Geometry check sheet. Reference: the model listing, model coordinates, mm. Face numbers are marked on the shaded views. Round coordinates to 2 decimals unless told otherwise and drop trailing zeros. Write each loop counter-clockwise with the first axis right and the second up, starting at its lowest first coordinate (ties: lowest second). Pieces come first, ordered by that corner, then holes. Notation, with made-up numbers: M -8,-3.75 L -2,-3.75 A28 cw -2,33.25 Z; hole C -23.5,15 d1. An arc over 180 degrees is marked long. Put each result on its own line as item: value. Start each with the question number.
(1) Section check D-D on y = 37. Record the cut outline in (x, z), then the cut area to 3 significant figures.
(2) Section check C-C on z = 2.7. Record the cut outline in (x, y), then the cut area to 3 significant figures.
(3) Material ranges on probe 1 along Y at (x, z) = (0, 3.95); probe 2 along X at (y, z) = (1.5, 2.4); probe 3 along X at (y, z) = (54, 0.5), recorded low to high.
(4) Section check A-A on y = 0. Record the cut outline in (x, z), then the cut area to 3 significant figures.
(5) Mould release check, pull along Z, two halves, no side actions. Record for the marked faces 1 and 2: pulls with the +Z half, pulls with the -Z half, needs draft (parallel to the pull), parting line crosses it, or undercut.
(6) Section check B-B on x = 0. Record the cut outline in (y, z), then the cut area to 3 significant figures.
(7) Gauge pin test, flat ends, axial feed: pin 1 (2 mm diameter, centred on y = 5.5, z = 3.5, fed in from +X); pin 2 (8 mm diameter, centred on x = 0, y = 0, fed in from +Z); pin 3 (1.2 mm diameter, centred on x = 0.5, z = 3, fed in from -Y); pin 4 (1.5 mm diameter, centred on y = 11, z = 0.5, fed in from -X). Record the tip position at first contact, or that the pin passes through.
from build123d import *

# Parameters (mm, degrees)
IZIM1_R                     = 63
Y_KSEKLIK_EKSTR_ZYON1_DEPTH = 5
IZIM2_R                     = 5
KES_EKSTR_ZYON1_DEPTH       = 10
IZIM3_W                     = 4
IZIM3_H                     = 4
KES_EKSTR_ZYON2_DEPTH       = 8


with BuildPart() as part:
    # Çizim1 → Yükseklik-Ekstrüzyon1 (new body)
    with BuildSketch(Plane.XY):
        Circle(IZIM1_R)
    extrude(amount=Y_KSEKLIK_EKSTR_ZYON1_DEPTH)

    # Çizim2 → Kes-Ekstrüzyon1 (cut)
    with BuildSketch(Plane.XY.offset(5)):
        Circle(IZIM2_R)
    extrude(amount=-KES_EKSTR_ZYON1_DEPTH, mode=Mode.SUBTRACT)

    # Çizim3 → Kes-Ekstrüzyon2 (cut)
    with BuildSketch(Plane(origin=(0, 0, 0), x_dir=(-1, 0, 0), z_dir=(0, 0, -1))):
        with Locations((0, 6.582575695)):
            Rectangle(IZIM3_W, IZIM3_H)
    extrude(amount=-KES_EKSTR_ZYON2_DEPTH, mode=Mode.SUBTRACT)


solid = part.part
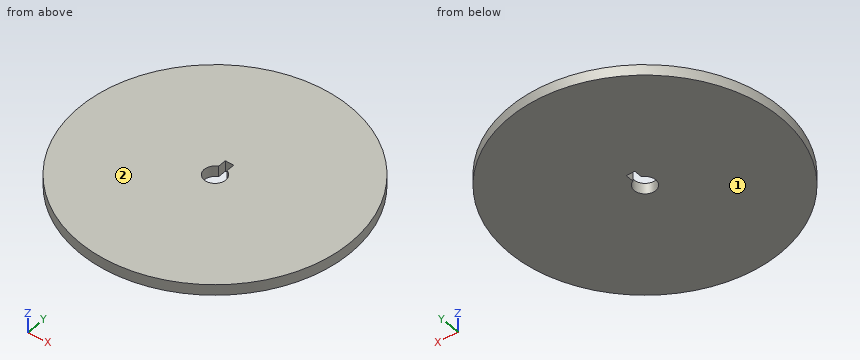
Answers follow:
1. outline: M -50.99,0 L 50.99,0 L 50.99,5 L -50.99,5 Z
1. area: 510 mm^2
2. outline: C 0,0 d126; hole M -2,4.58 A5 ccw long 2,4.58 L 2,8.58 L -2,8.58 Z
2. area: 12,400 mm^2
3. probe 1: y = -63 to -5, 8.58 to 63
3. probe 2: x = -62.98 to -4.77, 4.77 to 62.98
3. probe 3: x = -32.45 to 32.45
4. outline: M -63,0 L -5,0 L -5,5 L -63,5 Z; M 5,0 L 63,0 L 63,5 L 5,5 Z
4. area: 580 mm^2
5. face 1: pulls with the -Z half
5. face 2: pulls with the +Z half
6. outline: M -63,0 L -5,0 L -5,5 L -63,5 Z; M 8.58,0 L 63,0 L 63,5 L 8.58,5 Z
6. area: 562 mm^2
7. pin 1: stops at x = 62.84
7. pin 2: passes through
7. pin 3: stops at y = -63
7. pin 4: stops at x = -62.16
